CAD build for the part. Positions are in the model's coordinates, mm. Give positions to 0.01 mm unless a question says otherwise; leave off trailing zeros. Order: outer loops, then holes, each group sorted by start corner. A loop starts at its lowest first (then second) coordinate and runs counter-clockwise, first axis right, second up. Notation, with made-up numbers: (47.25, 53.25) -> (83.25, 53.25) arc R16 ccw to (83.25, 81.25) -> close; hole circle Ø6 at (80, 16). An arc over 180 degrees is marked (long way). Use one line per item in the form item = value. Start each with the question number.
1) Probe line 1 (Y direction, x = 1.1, z = 0) (1 decimal); line 2 (Y direction, x = 1.55, z = 2.25); line 3 (Y direction, x = 0.6, z = 7.25). List the from-to ranges inside material, lowest first.
2) Cut at C-C, the plane z = -5.5. Give the cut face in (x, y), and give its area (3 significant figures).
3) Cut at D-D, the plane y = 101.6. Give the cut face in (x, z), and give its area (3 significant figures).
4) Cut at B-B, the plane x = 1.1. State how many separate pieces and enclosed holes the cut face has, and give its area (3 significant figures).
5) Cut at A-A, the plane z = 0. Give the cut face in (x, y) (1 decimal).
from build123d import *

# Parameters (mm, degrees)
SKETCH1_R               = 11.1125
BOSS_EXTRUDE1_DEPTH     = 1.5875
F_1_4_CLEARANCE_HOLE1_D = 6.5278
M8_CLEARANCE_HOLE1_D    = 8.4


with BuildPart() as part:
    # Sketch1 → Boss-Extrude1 (new body)
    with BuildSketch(Plane(origin=(0, 0, 0), x_dir=(0, 0, -1), z_dir=(1, 0, 0))):
        with BuildLine():
            Line((9.518300378, 127.3571875), (12.134325567, 57.645583519))
            Line((12.134325567, 57.645583519), (10.547942171, 57.586052269))
            Line((10.547942171, 57.586052269), (11.738567171, 25.858384342))
            Line((11.738567171, 25.858384342), (13.324950567, 25.917915592))
            Line((13.324950567, 25.917915592), (14.277450567, 0.53578125))
            ThreePointArc((14.277450567, 0.53578125), (-0.331752192, -14.283647879), (-14.237180291, 1.198062439))
            Line((-14.237180291, 1.198062439), (-12.107291511, 26.508605179))
            Line((-12.107291511, 26.508605179), (-10.52538259, 26.37548713))
            Line((-10.52538259, 26.37548713), (-7.863021614, 58.013665555))
            Line((-7.863021614, 58.013665555), (-9.444930535, 58.146783604))
            Line((-9.444930535, 58.146783604), (-7.84751395, 77.129690658))
            ThreePointArc((-7.84751395, 77.129690658), (-7.764904905, 78.669797764), (-7.775922348, 80.212079439))
            Line((-7.775922348, 80.212079439), (-9.518300378, 126.6428125))
            ThreePointArc((-9.518300378, 126.6428125), (-0.3571875, 136.518300378), (9.518300378, 127.3571875))
        make_face()
        Circle(SKETCH1_R, mode=Mode.SUBTRACT)
    extrude(amount=BOSS_EXTRUDE1_DEPTH)

    # 1/4 Clearance Hole1 (through all)
    with Locations(Plane(origin=(1.5875, 0, 0), x_dir=(0, 0, -1), z_dir=(1, 0, 0))):
        with Locations((0, 127)):
            Hole(F_1_4_CLEARANCE_HOLE1_D / 2)

    # M8 Clearance Hole1 (through all)
    with Locations(Plane(origin=(1.5875, 0, 0), x_dir=(0, 0, -1), z_dir=(1, 0, 0))):
        with Locations((0, 101.6)):
            Hole(M8_CLEARANCE_HOLE1_D / 2)


solid = part.part
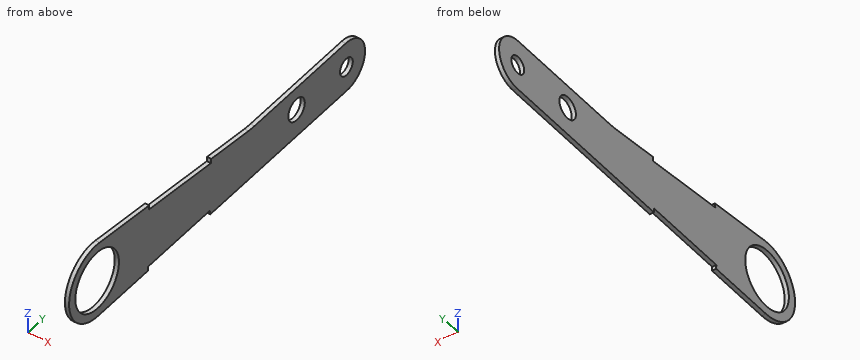
Result:
q1.line_1 = -14.3 to -11.1, 11.1 to 97.4, 105.8 to 123.7, 130.3 to 136.5
q1.line_2 = -14.11 to -10.88, 10.88 to 98.05, 105.15 to 124.64, 129.36 to 136.26
q1.line_3 = -12.31 to -8.42, 8.42 to 133.18
q2.outline = (0, -13.19) -> (1.59, -13.19) -> (1.59, -9.66) -> (0, -9.66) -> close; (0, 9.66) -> (1.59, 9.66) -> (1.59, 134.78) -> (0, 134.78) -> close
q2.area = 204 mm²
q3.outline = (0, -10.48) -> (1.59, -10.48) -> (1.59, -4.2) -> (0, -4.2) -> close; (0, 4.2) -> (1.59, 4.2) -> (1.59, 8.58) -> (0, 8.58) -> close
q3.area = 16.9 mm²
q4.separate_pieces = 1
q4.enclosed_holes = 3
q4.area = 2,680 mm²
q5.outline = (0, -14.3) -> (1.6, -14.3) -> (1.6, -11.1) -> (0, -11.1) -> close; (0, 11.1) -> (1.6, 11.1) -> (1.6, 97.4) -> (0, 97.4) -> close; (0, 105.8) -> (1.6, 105.8) -> (1.6, 123.7) -> (0, 123.7) -> close; (0, 130.3) -> (1.6, 130.3) -> (1.6, 136.5) -> (0, 136.5) -> close
